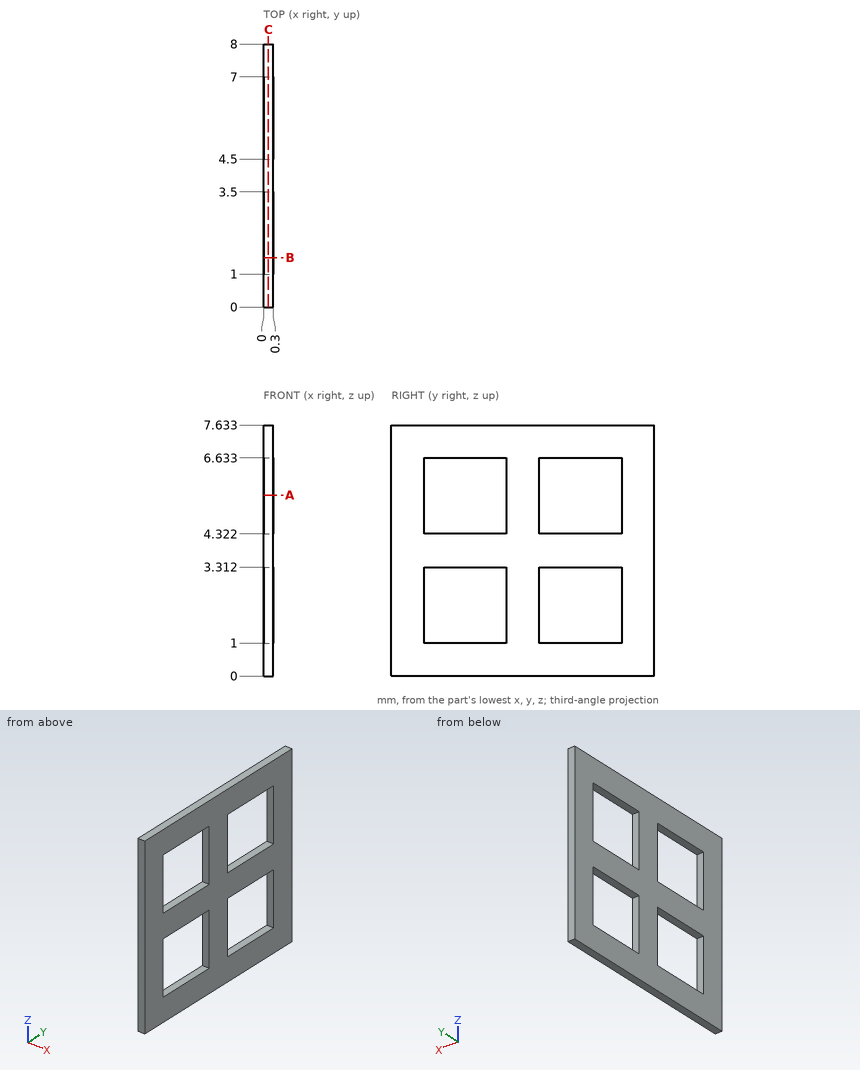
Source: three-view drawing plus pictorial views. Frame: mm from the lowest corner of the part. Give positions to 0.01 mm unless a question says otherwise; leave off trailing zeros. Loops run counter-clockwise (first coordinate to the right, second up) from the corner with the lowest first, then second, coordinate; pieces in that order, holes last.
1) Section query B-B on y = 1.5. Return the cut outline in (x, z).
A:
outline: (0, 0) - (0.3, 0) - (0.3, 1) - (0, 1) - close; (0, 3.31) - (0.3, 3.31) - (0.3, 4.32) - (0, 4.32) - close; (0, 6.63) - (0.3, 6.63) - (0.3, 7.63) - (0, 7.63) - close
2) Line query: L1, parallel to Y at x = 0.2, z = 5; L2, parallel to Z at x = 0.2, y = 5.5. Output: solid intervals per line, ascending.
A:
L1: y = 0 to 1, 3.5 to 4.5, 7 to 8
L2: z = 0 to 1, 3.31 to 4.32, 6.63 to 7.63
3) Section query C-C on x = 0.15. Return the cut outline in (y, z).
A:
outline: (0, 0) - (8, 0) - (8, 7.63) - (0, 7.63) - close; hole (1, 1) - (3.5, 1) - (3.5, 3.31) - (1, 3.31) - close; hole (1, 4.32) - (3.5, 4.32) - (3.5, 6.63) - (1, 6.63) - close; hole (4.5, 1) - (7, 1) - (7, 3.31) - (4.5, 3.31) - close; hole (4.5, 4.32) - (7, 4.32) - (7, 6.63) - (4.5, 6.63) - close
4) Section query A-A on z = 5.5. Return the cut outline in (x, y).
A:
outline: (0, 0) - (0.3, 0) - (0.3, 1) - (0, 1) - close; (0, 3.5) - (0.3, 3.5) - (0.3, 4.5) - (0, 4.5) - close; (0, 7) - (0.3, 7) - (0.3, 8) - (0, 8) - close
